Verification items for the finished model (mm, model axes). Face numbers are marked on the shaded views. A direction names the side the tool comes from. Coordinates: 2 decimals unless noted, no trailing zeros. Write each loop counter-clockwise with the first axis right and the second up, starting at its lowest first coordinate (ties: lowest second). Pieces come first, ordered by that corner, then holes. Notation, with made-up numbers: (50.5, 9) -> (56.5, 9) arc R31 cw to (56.5, 38) -> close; hole circle Ø9 at (89.25, 29). An arc over 180 degrees is marked (long way). Answer in a Markdown table with one row per item.
```python
from build123d import *

# Parameters (mm, degrees)
EXTRUDE_1_DEPTH     = 6
SKETCH_2_R          = 5.5
EXTRUDE_2_DEPTH     = 12
SKETCH_3_R          = 3
CUT_EXTRUDE_1_DEPTH = 13
SKETCH_4_R          = 2
CUT_EXTRUDE_2_DEPTH = 5
SKETCH_5_R          = 1.5
CUT_EXTRUDE_3_DEPTH = 12


with BuildPart() as part:
    # 草图1 → 凸台-拉伸1 (new body)
    with BuildSketch(Plane.XY):
        Polygon((6.92820323, 0), (3.464101615, 6), (-3.464101615, 6), (-6.92820323, 0), (-3.464101615, -6), (3.464101615, -6), align=None)
    extrude(amount=EXTRUDE_1_DEPTH)

    # 草图2 → 凸台-拉伸2 (add)
    with BuildSketch(Plane.XY.offset(6)):
        Circle(SKETCH_2_R)
    extrude(amount=EXTRUDE_2_DEPTH)

    # 草图3 → 切除-拉伸1 (cut)
    with BuildSketch(Plane.XY.offset(18)):
        Circle(SKETCH_3_R)
    extrude(amount=-CUT_EXTRUDE_1_DEPTH, mode=Mode.SUBTRACT)

    # 草图4 → 切除-拉伸2 (cut)
    with BuildSketch(Plane(origin=(0, 0, 0), x_dir=(-1, 0, 0), z_dir=(0, 0, -1))):
        Circle(SKETCH_4_R)
    extrude(amount=-CUT_EXTRUDE_2_DEPTH, mode=Mode.SUBTRACT)

    # 草图5 → 切除-拉伸3 (cut)
    with BuildSketch(Plane(origin=(0, 0, 0), x_dir=(1, 0, 0), z_dir=(0, 1, 0))):
        with Locations(Location((0, -13, 0), (0, 0, 90))):
            Circle(SKETCH_5_R)
    extrude(amount=CUT_EXTRUDE_3_DEPTH, mode=Mode.SUBTRACT)


solid = part.part
```
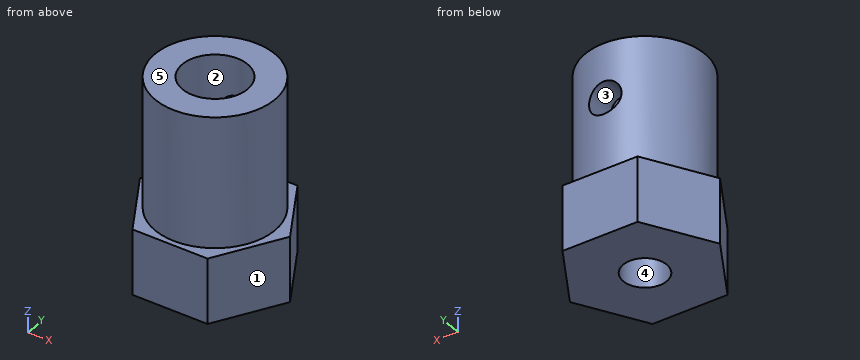
1. Go/stop test with flat-tipped pins: pin 1 (6 mm diameter, centred on y = 3.5, z = 15.5, fed in from -X); pin 2 (3 mm diameter, centred on x = -1, y = -1.5, fed in from +Z); pin 3 (3 mm diameter, centred on x = 0, y = 0, fed in from +Z); pin 4 (5 mm diameter, centred on y = -3.5, z = 11.5, fed in from +X). Record where each tip stops, or that it passes through.
Findings below:
| item | result |
|---|---|
| pin 1 | stops at x = -5.48 |
| pin 2 | stops at z = 18 |
| pin 3 | passes through |
| pin 4 | stops at x = 5.41 |
2. Sectioned sample at B-B, the plane z = 7. Record the cut outline in (x, y), and give its area (3 significant figures).
Findings below:
| item | result |
|---|---|
| outline | circle Ø11 at (0, 0); hole circle Ø6 at (0, 0) |
| area | 66.8 mm² |
3. Sectioned sample at D-D, the plane x = 5. Record the cut outline in (y, z).
Findings below:
| item | result |
|---|---|
| outline | (-3.34, 0) -> (3.34, 0) -> (3.34, 6) -> (2.29, 6) -> (2.29, 18) -> (-2.29, 18) -> (-2.29, 6) -> (-3.34, 6) -> close |
4. Release check for a two-part mould opening along Z. For the marked faces 3, 4 and 5 record: released by +Z, released by -Z, zero draft, split by the parting line, or undercut.
Findings below:
| item | result |
|---|---|
| face 3 | undercut |
| face 4 | zero draft |
| face 5 | released by +Z |
5. Material ranges on probe 1 along Y at (x, z) = (0, 8.5); probe 2 along Y at (x, z) = (0, 3.95); probe 3 along Z at (x, y) = (-0.5, 3.25), recorded low to high. Write a range as from..to.
Findings below:
| item | result |
|---|---|
| probe 1 | y = -5.5..-3, 3..5.5 |
| probe 2 | y = -6..-2, 2..6 |
| probe 3 | z = 0..11.59, 14.41..18 |
6. Sectioned sample at C-C, the plane y = -5. Record the cut outline in (x, z), and give its area (3 significant figures).
Findings below:
| item | result |
|---|---|
| outline | (-4.04, 0) -> (4.04, 0) -> (4.04, 6) -> (2.29, 6) -> (2.29, 18) -> (-2.29, 18) -> (-2.29, 6) -> (-4.04, 6) -> close |
| area | 103 mm² |
7. Access from +Z, -Z, +X, -X, +Y, -Y to the whole of each face (thin tool, end or side, straight path). Record for the marked faces 1 and 2.
Findings below:
| item | result |
|---|---|
| face 1 | +Z, -Z, +X, -Y |
| face 2 | +Z |
8. Sectioned sample at A-A, the plane x = 0. Record the cut outline in (y, z), and give its area (3 significant figures).
Findings below:
| item | result |
|---|---|
| outline | (-6, 0) -> (-2, 0) -> (-2, 5) -> (-3, 5) -> (-3, 18) -> (-5.5, 18) -> (-5.5, 6) -> (-6, 6) -> close; (2, 0) -> (6, 0) -> (6, 6) -> (5.5, 6) -> (5.5, 11.5) -> (3, 11.5) -> (3, 5) -> (2, 5) -> close; (3, 14.5) -> (5.5, 14.5) -> (5.5, 18) -> (3, 18) -> close |
| area | 98.5 mm² |
